```python
from build123d import *

# Parameters (mm, degrees)
SKETCH1_W           = 60
SKETCH1_H           = 13
BOSS_EXTRUDE1_DEPTH = 8
FILLET1_R           = 4
SKETCH2_W           = 20
SKETCH2_H           = 7
CUT_EXTRUDE1_DEPTH  = 32.721443851
SKETCH3_R           = 2
CUT_EXTRUDE2_DEPTH  = 34.660065359
SKETCH4_R           = 2
CUT_EXTRUDE3_DEPTH  = 32.721443851


with BuildPart() as part:
    # Sketch1 → Boss-Extrude1 (new body)
    with BuildSketch(Plane.XY):
        Rectangle(SKETCH1_W, SKETCH1_H)
    extrude(amount=BOSS_EXTRUDE1_DEPTH)

    # Fillet1
    fillet1_edges = [part.edges().sort_by_distance(p)[0] for p in [
        (-30, 0, 0),
        (30, 0, 0),
        (30, 0, 8),
        (-30, 0, 8),
    ]]
    fillet(fillet1_edges, radius=FILLET1_R - 0.0001)  # a hair under: the kernel refuses the full size

    # Sketch2 → Cut-Extrude1 (cut, through all)
    with BuildSketch(Plane.XY.offset(8)):
        with Locations((-20, 0)):
            Rectangle(SKETCH2_W, SKETCH2_H)
        with Locations((20, 0)):
            Rectangle(SKETCH2_W, SKETCH2_H)
    extrude(amount=-CUT_EXTRUDE1_DEPTH, mode=Mode.SUBTRACT)

    # Sketch3 → Cut-Extrude2 (cut, through all)
    with BuildSketch(Plane(origin=(0, 6.5, 0), x_dir=(1, 0, 0), z_dir=(0, 1, 0))):
        with Locations(Location((-22.5, -4, 0), (0, 0, 270))):
            Circle(SKETCH3_R)
        with Locations(Location((22.5, -4, 0), (0, 0, 270))):
            Circle(SKETCH3_R)
    extrude(amount=-CUT_EXTRUDE2_DEPTH, mode=Mode.SUBTRACT)

    # Sketch4 → Cut-Extrude3 (cut, through all)
    with BuildSketch(Plane.XY.offset(8)):
        Circle(SKETCH4_R)
    extrude(amount=-CUT_EXTRUDE3_DEPTH, mode=Mode.SUBTRACT)


solid = part.part
```
The model under review builds one solid part; all positions refer to its coordinate system, in mm. A direction names the side the tool comes from. Give positions to 0.01 mm unless a question says otherwise; leave off trailing zeros. Order: outer loops, then holes, each group sorted by start corner. A loop starts at its lowest first (then second) coordinate and runs counter-clockwise, first axis right, second up. Notation, with made-up numbers: (6.25, -31.75) - (39.25, -31.75) arc R20 ccw to (39.25, -11.75) - close; hole circle Ø7 at (-14, 38). An arc over 180 degrees is marked (long way). Use CSV: the item, a comma, the result in double quotes. Start each with the question number.
Q1. Clearance check with flat-ended pins moving along their axes: pin 1 Ø2 at (y, z) = (-1.5, 2.5) entering from -X; pin 2 Ø2 at (y, z) = (3, 1) entering from +X; pin 3 Ø2 at (y, z) = (0.5, 4.5) entering from +X. State where each tip first meets the part, or that it passes through.
Q2. To check wall thickness, follow line 1 along X through (y, z) = (-4.8, 4); line 2 along Y through (x, z) = (-11.5, 2); line 3 along Y through (x, z) = (0, 6.25). State the ranges of each line that lie inside material, in increasing order. Write a range as [from, to].
Q3. We need section C-C, the plane y = 0. Write out the cut boundary in (x, z), and give its area (3 significant figures).
Q4. We need section B-B, the plane z = 3.25. State how many separate pieces and enclosed holes the cut face has, and give its area (3 significant figures).
Q5. We need section D-D, the plane x = -24. Write out the cut boundary in (y, z), and give its area (3 significant figures).
Q6. Tool access review of faces 1 (the flat face through (0, -6.5, 4)), 2 (the flat face through (20, 3.5, 4)), 3 (the flat face through (-20, -3.5, 4)): name each direction out of +Z, -Z, +X, -X, +Y, -Y from which nothing blocks a thin tool from reaching the whole face with its end or side.
Q7. We need section A-A, the plane x = 25.5. Write out the cut boundary in (y, z).
Q8. The part is to be moulded in two halves that separate along Y. For faces 4 (the flat face through (0, 6.5, 4)), 5 (the cylindrical face through (21.3, -5, 2.4)), 6 (the flat face through (20, -3.5, 4)), say which applies: +Y half, -Y half, draft (parallel to the pull), parting line (faces both ways), or undercut.
Outcome:
1,pin 1,"stops at x = -10"
1,pin 2,"stops at x = 29.38"
1,pin 3,"stops at x = 10"
2,line 1,"x = [-30, -24.5], [-20.5, 20.5], [24.5, 30]"
2,line 2,"y = [-6.5, -3.5], [3.5, 6.5]"
2,line 3,"y = [-6.5, -2], [2, 6.5]"
3,outline,"(-10, 0) - (-2, 0) - (-2, 8) - (-10, 8) - close; (2, 0) - (10, 0) - (10, 8) - (2, 8) - close"
3,area,"128 mm^2"
4,separate pieces,"5"
4,enclosed holes,"1"
4,area,"442 mm^2"
5,outline,"(-6.5, 0) - (-3.5, 0) - (-3.5, 2.68) - (-6.5, 2.68) - close; (-6.5, 5.32) - (-3.5, 5.32) - (-3.5, 8) - (-6.5, 8) - close; (3.5, 0) - (6.5, 0) - (6.5, 2.68) - (3.5, 2.68) - close; (3.5, 5.32) - (6.5, 5.32) - (6.5, 8) - (3.5, 8) - close"
5,area,"32.1 mm^2"
6,face 1,"+Z, -Z, +X, -X, -Y"
6,face 2,"+Z, -Z, +X"
6,face 3,"+Z, -Z, -X"
7,outline,"(-6.5, 0) - (-3.5, 0) - (-3.5, 8) - (-6.5, 8) - close; (3.5, 0) - (6.5, 0) - (6.5, 8) - (3.5, 8) - close"
8,face 4,"+Y half"
8,face 5,"draft"
8,face 6,"undercut"
